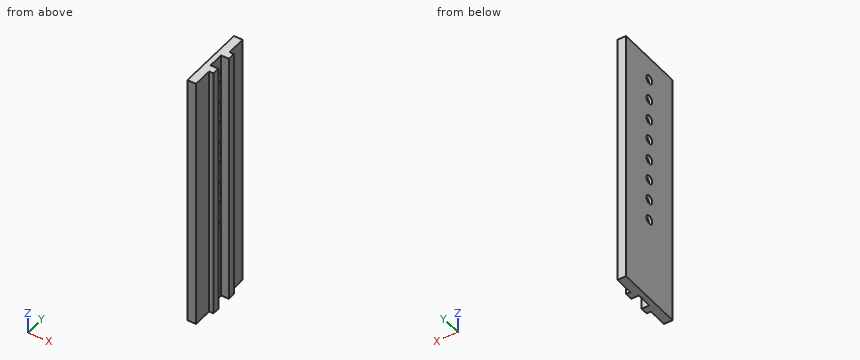
Autodesk Inventor part; units mm, degrees
ref_plane "YZ Plane" through (0, 0, 0) normal (1, 0, 0) x (0, 1, 0)
ref_plane "XZ Plane" through (0, 0, 0) normal (0, 1, 0) x (-1, 0, 0)
ref_plane "XY Plane" through (0, 0, 0) normal (0, 0, 1) x (1, 0, 0)
sketch "Sketch1" plane through (0, 0, 0) normal (0, 1, 0) x (-1, 0, 0)
  line L0 (0, 279.3478) -> (-39.1304, 279.3478)
  line L1 (-39.1304, 279.3478) -> (-39.1304, -320.6522)
  line L2 (-39.1304, -320.6522) -> (0, -320.6522)
  line L3 (0, -320.6522) -> (0, 279.3478)
  line L4 (-39.1304, 279.3478) -> (-29.1304, 279.3478)
  line L5 (-29.1304, 254.3478) -> (-39.1304, 254.3478)
  line L6 (-39.1304, 254.3478) -> (-39.1304, 279.3478)
  line L7 (-39.1304, -320.6522) -> (-29.1304, -320.6522)
  line L8 (-29.1304, -295.6522) -> (-39.1304, -295.6522)
  line L9 (-39.1304, -295.6522) -> (-39.1304, -320.6522)
  point P0 (0, 0)
  point P1 (-39.1304, 254.3478)
  point P2 (-39.1304, -295.6522)
  dimension "d0" = 600
  dimension "d4" = 25
  dimension "d5" = 25
  dimension "d28" = 39.1304
extrude "Extrusion1" add sketch "Sketch1" along normal blind 160
sketch "Sketch2" plane through (0, 0, 279.3478) normal (0, 0, 1) x (1, 0, 0)
  line L0 (0, 160) -> (39.1304, 160)
  line L1 (0, 160) -> (39.1304, 160)
  line L2 (39.1304, 160) -> (39.1304, 0)
  line L3 (39.1304, 0) -> (0, 0)
  line L4 (0, 0) -> (0, 160)
  line L5 (39.1304, 160) -> (29.1304, 160)
  line L6 (29.1304, 160) -> (29.1304, 115)
  line L7 (29.1304, 115) -> (39.1304, 115)
  line L8 (39.1304, 115) -> (39.1304, 160)
  line L9 (39.1304, 0) -> (29.1304, 0)
  line L10 (29.1304, 0) -> (29.1304, 45)
  line L11 (29.1304, 45) -> (39.1304, 45)
  line L12 (39.1304, 45) -> (39.1304, 0)
  circle A0 centre (39.1304, 80) radius 18
  line L13 (21.1304, 75) -> (39.1304, 75)
  line L14 (39.1304, 75) -> (39.1304, 98)
  line L15 (39.1304, 98) -> (21.1304, 98)
  line L16 (21.1304, 98) -> (21.1304, 75)
  line L17 (21.1304, 75) -> (39.1304, 75)
  line L18 (39.1304, 75) -> (39.1304, 62)
  line L19 (39.1304, 62) -> (21.1304, 62)
  line L20 (21.1304, 62) -> (21.1304, 75)
  line L21 (39.1304, 0) -> (39.1304, 160)
  line L22 (0, 160) -> (9.1304, 160)
  line L23 (9.1304, 160) -> (9.1304, 0)
  line L24 (9.1304, 0) -> (0, 0)
  line L25 (0, 0) -> (0, 160)
  point P0 (0, 0)
  point P1 (34.1304, 115)
  point P2 (34.1304, 160)
  point P3 (39.1304, 45)
  point P4 (39.1304, 115)
  dimension "d6" = 10
  dimension "d7" = 45
  dimension "d8" = 45
  dimension "d9" = 18
  dimension "d10" = 36
  dimension "d11" = 80
  dimension "d12" = 80
  dimension "d15" = 30
extrude "Extrusion2" cut sketch "Sketch2" against normal up to surface (600 mm away) contours L0 L23 L3 L4 | L0 L2 L7 L6 | L10 L11 L2 L3 | L2 L13 A0 | A0 L16 L15 | L2 A0 L13 | A0 L13 L16 | L19 L20 L13 A0
sketch "Sketch3" plane through (21.1304, 62, 279.3478) normal (1, 0, 0) x (0, 0, -1)
  line L0 (600, 0) -> (0, 0)
  line L1 (0, 0) -> (0, 36)
  line L2 (0, 36) -> (600, 36)
  circle A0 centre (54, 18) radius 10
  circle A1 centre (104, 18) radius 10
  circle A2 centre (154, 18) radius 10
  circle A3 centre (204, 18) radius 10
  circle A4 centre (254, 18) radius 10
  circle A5 centre (304, 18) radius 10
  circle A6 centre (354, 18) radius 10
  circle A7 centre (404, 18) radius 10
  circle A8 centre (454, 18) radius 10
  point P0 (279.3478, -62)
  dimension "d18" = 50
extrude "Extrusion3" cut sketch "Sketch3" against normal blind 25 contours A0 | A1 | A2 | A3 | A4 | A5 | A6 | A7
chamfer "Chamfer1" distance 8 distance2 5 8 edges at (21.1304, 80, 235.3478) (21.1304, 80, 185.3478) (21.1304, 80, 135.3478) (21.1304, 80, 85.3478) (21.1304, 80, 35.3478) (21.1304, 80, -14.6522) (21.1304, 80, -64.6522) (21.1304, 80, -114.6522) measured on face at (21.1304, 80, -258.6522)
properties part number "MainRails" material "Aluminum 6061"
CAD build for the part. Positions are in the model's coordinates, mm. Round coordinates to 2 decimals unless told otherwise and drop trailing zeros. Loops run counter-clockwise (first coordinate to the right, second up) from the corner with the lowest first, then second, coordinate; pieces in that order, holes last. Notation, with made-up numbers: M 55.5,66.5 L 65.5,66.5 A22 ccw 65.5,105.5 Z; hole C 67.5,-32 d3. An arc over 180 degrees is marked long. Use a Markdown table: item, result. Add a question column.
(1) Cut at B-B (y = 80). State how many separate pieces and enclosed holes the cut face has, and give its area (3 significant figures).
(2) Cut at C-C (y = 145). Give the cut face in (x, z).
(3) Drill centre lines: line 1 (Y direction, x = 37, z = 7); line 2 (Y direction, x = 26.5, z = 166); line 3 (X direction, y = 23, z = -219). Where is each one in solid material? Low to high.
(4) Cut at A-A (z = 202). Give the cut face in (x, y), and give its area (3 significant figures).
(5) Flat gauge pins, fed straight in: pin 1 (13.5 mm diameter, centred on y = 27, z = 9.5, fed in from +X); pin 2 (5 mm diameter, centred on x = 20.5, z = -145, fed in from -Y); pin 3 (8 mm diameter, centred on x = 34.5, z = -84, fed in from -Y); pin 4 (5.5 mm diameter, centred on x = 32, z = 35.5, fed in from +Y). Where does each tip first touch, or does it go through?
Geometry says:
| question | item | result |
|---|---|---|
| 1 | separate pieces | 9 |
| 1 | enclosed holes | 0 |
| 1 | area | 4,960 mm² |
| 2 | outline | M 9.13,-320.65 L 29.13,-320.65 L 29.13,279.35 L 9.13,279.35 Z |
| 3 | line 1 | y = 45 to 62, 98 to 115 |
| 3 | line 2 | y = 0 to 62, 98 to 160 |
| 3 | line 3 | x = 9.13 to 29.13 |
| 4 | outline | M 9.13,0 L 29.13,0 L 29.13,45 L 39.13,45 L 39.13,62 L 21.13,62 L 21.13,98 L 39.13,98 L 39.13,115 L 29.13,115 L 29.13,160 L 9.13,160 Z |
| 4 | area | 3,250 mm² |
| 5 | pin 1 | stops at x = 29.13 |
| 5 | pin 2 | stops at y = 0 |
| 5 | pin 3 | stops at y = 45 |
| 5 | pin 4 | stops at y = 115 |
